```python
from build123d import *

# Parameters (mm, degrees)
SKETCH167_R      = 10
EXTRUDE147_DEPTH = 4
BODY018_W        = 39
BODY018_H        = 174
EXTRUDE_DEPTH    = 2


with BuildPart() as extrude147:
    # Sketch167 → Extrude147 (new body)
    with BuildSketch(Plane.XY.offset(29)):
        with Locations((211.272537, 288)):
            Circle(SKETCH167_R)
        with Locations((245.453842, 288)):
            Circle(SKETCH167_R)
        with Locations((279.504333, 288)):
            Circle(SKETCH167_R)
        with Locations((345.672821, 288)):
            Circle(SKETCH167_R)
        with Locations((313, 288)):
            Circle(SKETCH167_R)
    extrude(amount=-EXTRUDE147_DEPTH)


with BuildPart() as cut010:
    # Body018 → Extrude (new body)
    with BuildSketch(Plane(origin=(278, 287.5, 26), x_dir=(0, -1, 0), z_dir=(0, 0, -1))):
        Rectangle(BODY018_W, BODY018_H)
    extrude(amount=-EXTRUDE_DEPTH)

    # Cut010: cut Extrude147
    add(extrude147.part, mode=Mode.SUBTRACT)


solid = cut010.part
```
Input: part model. Units: mm. Frame: model coordinates. Round coordinates to 2 decimals unless told otherwise and drop trailing zeros. Loops run counter-clockwise (first coordinate to the right, second up) from the corner with the lowest first, then second, coordinate; pieces in that order, holes last. Notation, with made-up numbers: M -25.5,1.25 L 17.5,1.25 A16 ccw 17.5,27.25 Z; hole C 66,8 d6. An arc over 180 degrees is marked long. Answer in a Markdown table with one row per item. Add a question column.
1. Section B-B (x = 313). Output: boundary loops of the cut face in (y, z).
2. Mould query, pull axis Y, two halves, no side actions, for faces 1 (the face through (284.12, 279.13, 27.01)), 2 (the face through (277, 275, 26)), 3 (the face through (350.29, 279.13, 27.01)). Classes: released by +Y, released by -Y, zero draft, split by the parting line, or undercut.
3. Ray query, probe 1 along X at (y, z) = (281.5, 27.45) (1 decimal); probe 2 along X at (y, z) = (281, 26.55); probe 3 along Y at (x, z) = (274.5, 27.2). Return the intervals inside material, ascending.
4. Section A-A (y = 288). Output: boundary loops of the cut face in (x, z).
5. Section D-D (y = 281). Output: boundary loops of the cut face in (x, z), and give its area (3 significant figures).
6. Section C-C (z = 27.6). Output: boundary loops of the cut face in (x, y).
Values follow:
| question | item | result |
|---|---|---|
| 1 | outline | M 268,26 L 278,26 L 278,28 L 268,28 Z; M 298,26 L 307,26 L 307,28 L 298,28 Z |
| 2 | face 1 | undercut |
| 2 | face 2 | zero draft |
| 2 | face 3 | undercut |
| 3 | probe 1 | 191 to 203.7, 218.9 to 237.9, 253.1 to 271.9, 287.1 to 305.4, 320.6 to 338.1, 353.3 to 365 |
| 3 | probe 2 | 191 to 204.13, 218.41 to 238.31, 252.6 to 272.36, 286.65 to 305.86, 320.14 to 338.53, 352.81 to 365 |
| 3 | probe 3 | 268 to 279.34, 296.66 to 307 |
| 4 | outline | M 191,26 L 201.27,26 L 201.27,28 L 191,28 Z; M 221.27,26 L 235.45,26 L 235.45,28 L 221.27,28 Z; M 255.45,26 L 269.5,26 L 269.5,28 L 255.45,28 Z; M 289.5,26 L 303,26 L 303,28 L 289.5,28 Z; M 323,26 L 335.67,26 L 335.67,28 L 323,28 Z; M 355.67,26 L 365,26 L 365,28 L 355.67,28 Z |
| 5 | outline | M 191,26 L 204.13,26 L 204.13,28 L 191,28 Z; M 218.41,26 L 238.31,26 L 238.31,28 L 218.41,28 Z; M 252.6,26 L 272.36,26 L 272.36,28 L 252.6,28 Z; M 286.65,26 L 305.86,26 L 305.86,28 L 286.65,28 Z; M 320.14,26 L 338.53,26 L 338.53,28 L 320.14,28 Z; M 352.81,26 L 365,26 L 365,28 L 352.81,28 Z |
| 5 | area | 205 mm^2 |
| 6 | outline | M 191,268 L 365,268 L 365,307 L 191,307 Z; hole C 211.27,288 d20; hole C 245.45,288 d20; hole C 279.5,288 d20; hole C 313,288 d20; hole C 345.67,288 d20 |
